Build history of the part. All positions in model axes, mm. A direction names the side the tool comes from. Round coordinates to 2 decimals unless told otherwise and drop trailing zeros. Write each loop counter-clockwise with the first axis right and the second up, starting at its lowest first coordinate (ties: lowest second). Pieces come first, ordered by that corner, then holes. Notation, with made-up numbers: (60.25, 13) -> (105.25, 13) arc R21 ccw to (105.25, 17) -> close; hole circle Ø9 at (32, -32.5). An arc over 180 degrees is marked (long way). One line per question, with ' | ' between items.
from build123d import *

# Parameters (mm, degrees)
SKETCH1_W           = 23.7
SKETCH1_H           = 36.8
BOSS_EXTRUDE2_DEPTH = 46
SKETCH2_R           = 10
CUT_EXTRUDE1_DEPTH  = 5


with BuildPart() as part:
    # Sketch1 → Boss-Extrude2 (new body)
    with BuildSketch(Plane.XY):
        with Locations((-2.757896825, -4.218611111)):
            Rectangle(SKETCH1_W, SKETCH1_H)
    extrude(amount=BOSS_EXTRUDE2_DEPTH)

    # Sketch2 → Cut-Extrude1 (cut)
    with BuildSketch(Plane(origin=(0, 14.181388889, 0), x_dir=(1, 0, 0), z_dir=(0, 1, 0))):
        with Locations((-3.007896825, -34.4)):
            Circle(SKETCH2_R)
    cut_extrude1 = extrude(amount=-CUT_EXTRUDE1_DEPTH, mode=Mode.SUBTRACT)

    # Mirror1: Cut-Extrude1 across plane
    add(cut_extrude1.mirror(Plane.ZX.offset(-4.218611111)), mode=Mode.SUBTRACT)


solid = part.part
(1) Wall check: line 1 (X direction, y = 13.15, z = 34.4); line 2 (Y direction, x = -6.75, z = 32); line 3 (Z direction, x = -4.75, y = 10.5). Give the ranges that are in metal, low to high. Write a range as from..to.
Calculated:
line 1: -14.61..-13.01, 6.99..9.09 | line 2: -17.62..9.18 | line 3: 0..24.55, 44.25..46
(2) Slice it at C-C (x = -11). Write the cut outline in (y, z).
Calculated:
outline: (-22.62, 0) -> (14.18, 0) -> (14.18, 28.39) -> (9.18, 28.39) -> (9.18, 40.41) -> (14.18, 40.41) -> (14.18, 46) -> (-22.62, 46) -> (-22.62, 40.41) -> (-17.62, 40.41) -> (-17.62, 28.39) -> (-22.62, 28.39) -> close
(3) Drop flat-ended pins along their axis: pin 1 (6 mm diameter, centred on x = 0.5, z = 29.5, fed in from -Y); pin 2 (8 mm diameter, centred on x = 4, z = 36, fed in from +Y); pin 3 (6 mm diameter, centred on x = -6, z = 33.5, fed in from +Y). Give the stop position or say it passes through.
Calculated:
pin 1: y = -17.62 | pin 2: y = 14.18 | pin 3: y = 9.18
(4) Mould opens along Z. For faces 4 (the cylindrical face through (-4.31, 11.716, 24.485)), 5 (the flat face through (-3, -4, 46)), 6 (the flat face through (9.092, -4, 23)) say: pulls with the +Z half, pulls with the -Z half, needs draft (parallel to the pull), parting line crosses it, or undercut.
Calculated:
face 4: undercut | face 5: pulls with the +Z half | face 6: needs draft
(5) Slice it at B-B (y = 11). Write the cut outline in (x, z), then the cut area to 3 significant figures.
Calculated:
outline: (-14.61, 0) -> (9.09, 0) -> (9.09, 46) -> (-14.61, 46) -> close; hole circle Ø20 at (-3.01, 34.4) | area: 776 mm2
(6) 3-axis set-ups, long thin cutter, end or side, ignore diameter. For faces 1 (the flat face through (-3, -17.619, 34)), 2 (the flat face through (-3, -22.619, 18)), 3 (the flat face through (-3, 9.181, 34)): which of +Z, -Z, +X, -X, +Y, -Y reach the whole face in a straight line?
Calculated:
face 1: -Y | face 2: +Z, -Z, +X, -X, -Y | face 3: +Y
(7) Slice it at A-A (z = 34.4). Write the cut outline in (x, y), then the cut area to 3 significant figures.
Calculated:
outline: (-14.61, -22.62) -> (-13.01, -22.62) -> (-13.01, -17.62) -> (6.99, -17.62) -> (6.99, -22.62) -> (9.09, -22.62) -> (9.09, 14.18) -> (6.99, 14.18) -> (6.99, 9.18) -> (-13.01, 9.18) -> (-13.01, 14.18) -> (-14.61, 14.18) -> close | area: 672 mm2
